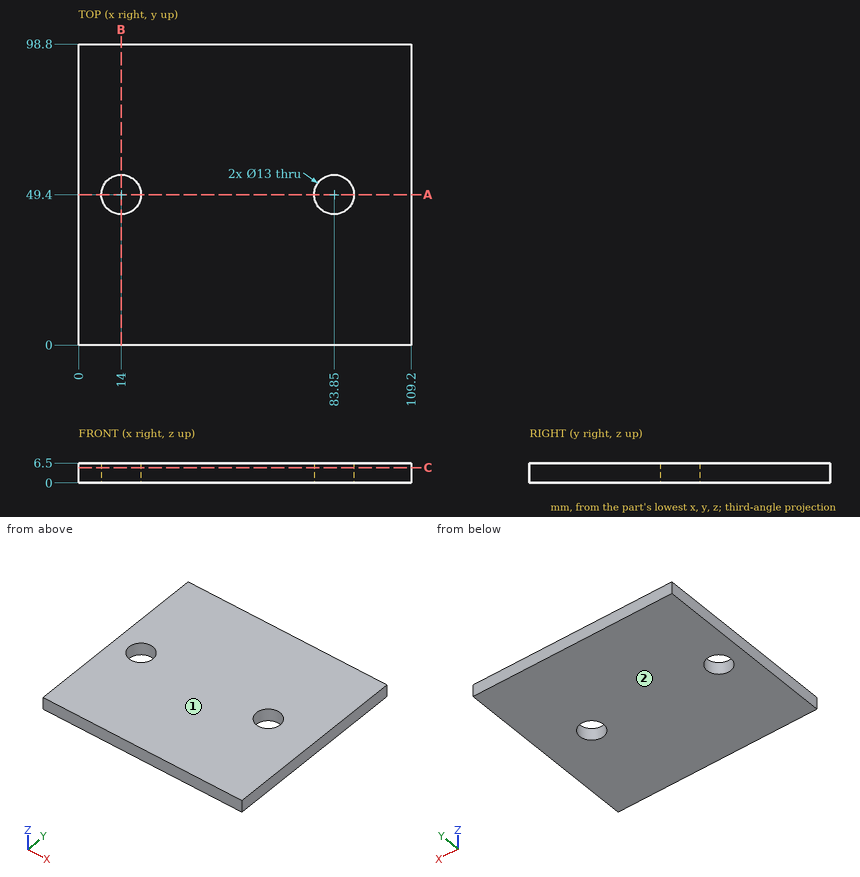
Geometry check sheet. Reference: drawing and pictorial views, mm from the part's lowest x, y, z. Give positions to 0.01 mm unless a question says otherwise; leave off trailing zeros. Order: outer loops, then holes, each group sorted by start corner. A loop starts at its lowest first (then second) coordinate and runs counter-clockwise, first axis right, second up. Notation, with made-up numbers: M 30.25,72.25 L 89.25,72.25 A20 cw 89.25,103.25 Z; hole C -24,43 d1. An arc over 180 degrees is marked long. Answer as a JSON object with one key per item and string values. Group by question number.
1) Cross-section at A-A (y = 49.4). Enter the section's corners in (x, z).
2) Scan lines: line 1 along X through (y, z) = (49.4, 2); line 2 along Y through (x, z) = (83.85, 3.5); line 3 along Y through (x, z) = (12, 2). Record each from-to range of solid material in increasing order. Write a range as [from, to].
3) Depth check by flat-ended pin: pin 1 Ø2 at (y, z) = (82.5, 4) entering from -X; pin 2 Ø11.5 at (x, y) = (14, 49.4) entering from -Z. Enter the tip coordinate at first touch or a pass-through.
4) Cross-section at C-C (z = 5). Enter the section's corners in (x, y).
5) Mould release check, pull along Z, two halves, no side actions. Record for the marked faces 1 and 2: released by +Z, released by -Z, zero draft, split by the parting line, or undercut.
6) Cross-section at B-B (x = 14). Enter the section's corners in (y, z).
Result sheet:
{
 "1": {"outline": "M 0,0 L 7.5,0 L 7.5,6.5 L 0,6.5 Z; M 20.5,0 L 77.35,0 L 77.35,6.5 L 20.5,6.5 Z; M 90.35,0 L 109.2,0 L 109.2,6.5 L 90.35,6.5 Z"},
 "2": {"line 1": "x = [0, 7.5], [20.5, 77.35], [90.35, 109.2]", "line 2": "y = [0, 42.9], [55.9, 98.8]", "line 3": "y = [0, 43.22], [55.58, 98.8]"},
 "3": {"pin 1": "stops at x = 0", "pin 2": "passes through"},
 "4": {"outline": "M 0,0 L 109.2,0 L 109.2,98.8 L 0,98.8 Z; hole C 14,49.4 d13; hole C 83.85,49.4 d13"},
 "5": {"face 1": "released by +Z", "face 2": "released by -Z"},
 "6": {"outline": "M 0,0 L 42.9,0 L 42.9,6.5 L 0,6.5 Z; M 55.9,0 L 98.8,0 L 98.8,6.5 L 55.9,6.5 Z"}
}
